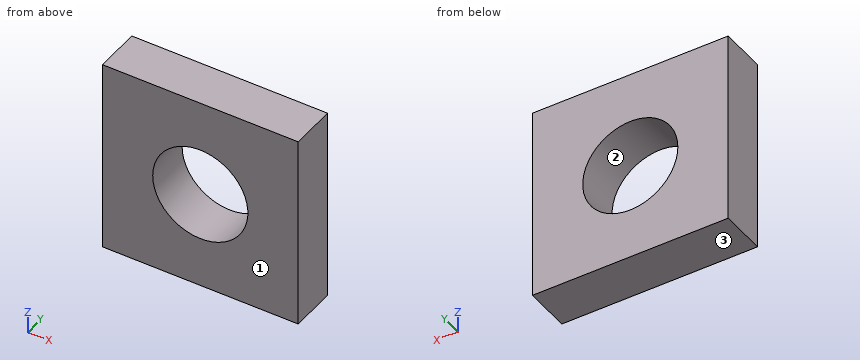
Autodesk Inventor part; units mm, degrees
sketch "スケッチ1" plane through (0, 0, 0) normal (0, 1, 0) x (-1, 0, 0)
  circle A0 centre (0, 0) radius 17.5
  line L0 (36, -36) -> (-36, -36)
  line L1 (-36, -36) -> (-36, 36)
  line L2 (-36, 36) -> (36, 36)
  line L3 (36, 36) -> (36, -36)
  line L4 (36, -36) -> (-36, 36) construction
  line L5 (-36, -36) -> (36, 36) construction
  dimension "d0" = 35
  dimension "d1" = 72
  dimension "d2" = 72
extrude "押し出し1" add sketch "スケッチ1" along normal blind 17
properties part number "bearing3b"
Source: CAD feature listing. Evaluate the final solid. Frame: model axes, mm. Face numbers are marked on the shaded views. Round coordinates to 2 decimals unless told otherwise and drop trailing zeros. Write each loop counter-clockwise with the first axis right and the second up, starting at its lowest first coordinate (ties: lowest second). Pieces come first, ordered by that corner, then holes. Notation, with made-up numbers: M -5.5,-33.5 L 51.5,-33.5 A32 cw 51.5,0.5 Z; hole C 46,77 d6. An arc over 180 degrees is marked long. One line per item, written item: value. Start each with the question number.
Item 1: Pin query (flat end, axial travel): pin 1 (8 mm diameter, centred on x = -27.5, z = -9.5, fed in from -Y). Return the tip coordinate at first contact, or that it passes through.
Item 2: Ray query, L1, parallel to Z at x = 0, y = 12.5; L2, parallel to X at y = 12, z = -8; L3, parallel to X at y = 9.5, z = -5. Return the intervals inside material, ascending. Write a range as from..to.
Item 3: Section query B-B (x = 0). Return the cut outline in (y, z).
Item 4: Mould query, pull axis Z, two halves, no side actions, for the marked faces 1, 2 and 3. Classes: pulls with the +Z half, pulls with the -Z half, needs draft (parallel to the pull), parting line crosses it, or undercut.
Item 5: Section query C-C (y = 12). Return the cut outline in (x, z), plus the area to 3 significant figures.
Item 6: Section query A-A (z = 0). Return the cut outline in (x, y).
Result set:
1. pin 1: stops at y = 0
2. L1: z = -36..-17.5, 17.5..36
2. L2: x = -36..-15.56, 15.56..36
2. L3: x = -36..-16.77, 16.77..36
3. outline: M 0,-36 L 17,-36 L 17,-17.5 L 0,-17.5 Z; M 0,17.5 L 17,17.5 L 17,36 L 0,36 Z
4. face 1: needs draft
4. face 2: undercut
4. face 3: pulls with the -Z half
5. outline: M -36,-36 L 36,-36 L 36,36 L -36,36 Z; hole C 0,0 d35
5. area: 4,220 mm²
6. outline: M -36,0 L -17.5,0 L -17.5,17 L -36,17 Z; M 17.5,0 L 36,0 L 36,17 L 17.5,17 Z
